Work out the finished part from the listing and answer in its coordinate system (mm). A direction names the side the tool comes from. Round coordinates to 2 decimals unless told otherwise and drop trailing zeros. Write each loop counter-clockwise with the first axis right and the second up, starting at its lowest first coordinate (ties: lowest second). Pieces come first, ordered by that corner, then holes.
from build123d import *

# Parameters (mm, degrees)
SKETCH1_R                               = 28
BOSS_EXTRUDE1_DEPTH                     = 50
SKETCH1_3_R                             = 125
BOSS_EXTRUDE2_DEPTH                     = 200
CBORE_FOR_M5_HEX_HEAD_BOLT1_D           = 125
CBORE_FOR_M5_HEX_HEAD_BOLT1_DEPTH       = 200
CBORE_FOR_M5_HEX_HEAD_BOLT1_CBORE_D     = 188
CBORE_FOR_M5_HEX_HEAD_BOLT1_CBORE_DEPTH = 50
CBORE_FOR_M5_HEX_HEAD_BOLT1_TIP         = 36.084391824


with BuildPart() as part:
    # Sketch1 → Boss-Extrude1 (new body)
    with BuildSketch(Plane(origin=(0, 0, 0), x_dir=(1, 0, 0), z_dir=(0, 1, 0))):
        with BuildLine():
            ThreePointArc((-125, -69), (-108.597979746, -108.597979746), (-69, -125))
            Line((-69, -125), (125, -125))
            ThreePointArc((125, -125), (0, 0), (125, 125))
            Line((125, 125), (-69, 125))
            ThreePointArc((-69, 125), (-108.597979746, 108.597979746), (-125, 69))
            Line((-125, 69), (-125, -69))
        make_face()
        with Locations(Location((-69, -69, 0), (0, 0, 270))):
            Circle(SKETCH1_R, mode=Mode.SUBTRACT)
        with Locations(Location((-69, 69, 0), (0, 0, 270))):
            Circle(SKETCH1_R, mode=Mode.SUBTRACT)
    extrude(amount=BOSS_EXTRUDE1_DEPTH)

    # Sketch1_3 → Boss-Extrude2 (add)
    with BuildSketch(Plane(origin=(0, 0, 0), x_dir=(1, 0, 0), z_dir=(0, 1, 0))):
        with Locations(Location((125, 0, 0), (0, 0, 270))):
            Circle(SKETCH1_3_R)
    extrude(amount=BOSS_EXTRUDE2_DEPTH)

    # CBORE for M5 Hex Head Bolt1
    with Locations(Plane(origin=(0, 200, 0), x_dir=(1, 0, 0), z_dir=(0, 1, 0))):
        with Locations((125, 0)):
            CounterBoreHole(CBORE_FOR_M5_HEX_HEAD_BOLT1_D / 2, CBORE_FOR_M5_HEX_HEAD_BOLT1_CBORE_D / 2, CBORE_FOR_M5_HEX_HEAD_BOLT1_CBORE_DEPTH, depth=CBORE_FOR_M5_HEX_HEAD_BOLT1_DEPTH)
            with Locations((0, 0, -(CBORE_FOR_M5_HEX_HEAD_BOLT1_DEPTH + CBORE_FOR_M5_HEX_HEAD_BOLT1_TIP / 2))):  # 120° drill point
                Cone(0, CBORE_FOR_M5_HEX_HEAD_BOLT1_D / 2, CBORE_FOR_M5_HEX_HEAD_BOLT1_TIP, mode=Mode.SUBTRACT)

    # Sketch7 → Loft1 section 0
    with BuildSketch(Plane(origin=(0, 50, 0), x_dir=(1, 0, 0), z_dir=(0, 1, 0))):
        with BuildLine():
            Line((-125, 22), (19.117040025, 22))
            Line((19.117040025, 22), (19.117040025, -22))
            Line((19.117040025, -22), (-125, -22))
            Line((-125, -22), (-125, 22))
        make_face()
    # Sketch6 for Loft1 → Loft1 section 1
    with BuildSketch(Plane(origin=(0, 200, 0), x_dir=(1, 0, 0), z_dir=(0, 1, 0))):
        with BuildLine():
            Line((1.951229181, -22), (26.938517531, -22))
            Line((26.938517531, -22), (26.938517531, 22))
            Line((26.938517531, 22), (1.951229181, 22))
            # circular arc as an exact rational Bezier (weights 1, cos(half-angle), 1)
            Bezier((1.951229181, 22), (-1.982170533, 0), (1.951229181, -22), weights=[1, 0.984390167, 1])
        make_face()
    loft()


solid = part.part
Q1. A tool of negligible diameter and unlimited length cuts with its end or side. For faces 1 (the face through (-30, 50, -74)), 2 (the face through (31.09, 175.35, -4.13)), 3 (the face through (-30, 50, 73)), from which of +Z, -Z, +X, -X, +Y, -Y can it reach the whole face along a straight path? Write none if from no direction.
Q2. Find section C-C (z = 26). Determine the outline of the cut face in (x, y).
Q3. Find section D-D (x = 212). Determine the outline of the cut face in (y, z), plus the area to 3 significant figures.
Q4. Given pin 1 (8 mm diameter, centred on y = 75.5, z = 51.5, fed in from +X); pin 2 (1.5 mm diameter, centred on y = 111.5, z = 52, fed in from -X); pin 3 (1.5 mm diameter, centred on y = 79, z = -40.5, fed in from +X), each flat-ended and moving along its own axis, determine where each tip first touches the part or whether it passes through.
Q5. Find section B-B (x = 164.5). Determine the outline of the cut face in (y, z).
Q6. Find section A-A (y = 13). Determine the outline of the cut face in (x, z), plus the area to 3 significant figures.
Q7. The mould has two halves that part along X. Classify faces 4 (the face through (27, 25, 125)), 5 (the face through (-108.16, 24.65, -109.03)), 6 (the face through (65.386, 73.95, -18.773)), 7 (the face through (-67.769, 24.65, 41.027)): +X half, -X half, draft (parallel to the pull), parting line (faces both ways), or undercut.
Q8. Find the intervals of material crossed by L1, parallel to X at y = 14, z = 63; L2, parallel to X at y = 105, z = -9.5; L3, parallel to Z at x = 125, y = 161, in increasing order.
Report:
1. face 1: -Z, -X, +Y
1. face 2: +Y
1. face 3: +Z, -X, +Y
2. outline: (-125, 0) - (68.16, 0) - (68.16, 150) - (34.67, 150) - (34.67, 200) - (2.73, 200) - (2.73, 50) - (-125, 50) - close; (181.84, 0) - (247.27, 0) - (247.27, 200) - (215.33, 200) - (215.33, 150) - (181.84, 150) - close
3. outline: (0, -89.76) - (200, -89.76) - (200, -35.59) - (150, -35.59) - (150, 35.59) - (200, 35.59) - (200, 89.76) - (0, 89.76) - close
3. area: 32,300 mm2
4. pin 1: stops at x = 240.62
4. pin 2: stops at x = 10.99
4. pin 3: stops at x = 243.51
5. outline: (0, -118.59) - (200, -118.59) - (200, -85.3) - (150, -85.3) - (150, -48.44) - (0, -48.44) - close; (0, 48.44) - (150, 48.44) - (150, 85.3) - (200, 85.3) - (200, 118.59) - (0, 118.59) - close
6. outline: (-125, -69) arc R56 ccw to (-69, -125) - (125, -125) arc R125 ccw to (125, 125) - (-69, 125) arc R56 ccw to (-125, 69) - close; hole circle Ø56 at (-69, -69); hole circle Ø56 at (-69, 69); hole circle Ø125 at (125, 0)
6. area: 68,500 mm2
7. face 4: draft
7. face 5: -X half
7. face 6: undercut
7. face 7: undercut
8. L1: x = -125 to -96.35, -41.65 to 232.96
8. L2: x = -79.03 to 63.23, 186.77 to 249.64
8. L3: z = -125 to -94, 94 to 125
